CAD build for the part. Positions are in the model's coordinates, mm. Face numbers are marked on the shaded views. A direction names the side the tool comes from. Coordinates: 2 decimals unless noted, no trailing zeros. Loops run counter-clockwise (first coordinate to the right, second up) from the corner with the lowest first, then second, coordinate; pieces in that order, holes last. Notation, with made-up numbers: (7.25, -14) -> (15.25, -14) arc R22 ccw to (15.25, 6) -> close; hole circle Ø8 at (18, -27). An arc over 180 degrees is marked (long way). Write each question's results on one line, items separated by ' | '.
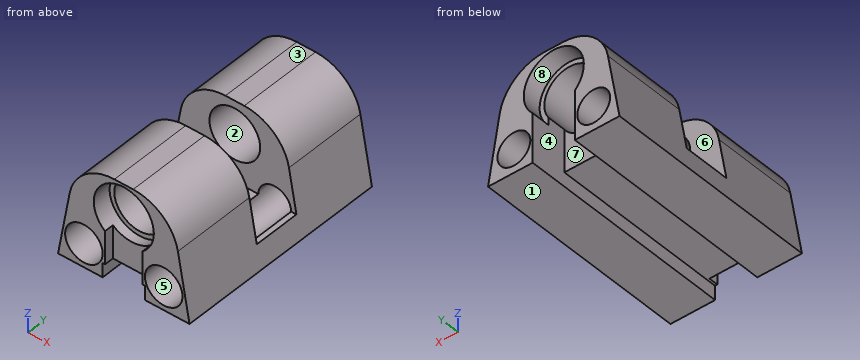
```python
from build123d import *

# Parameters (mm, degrees)
PAD_DEPTH       = 11.5
SKETCH001_W     = 14
SKETCH001_H     = 5
POCKET_DEPTH    = 8.5
SKETCH002_R     = 1.75
POCKET001_DEPTH = 23.001
SKETCH003_R     = 2.7
POCKET002_DEPTH = 23.001
SKETCH004_R     = 2
POCKET003_DEPTH = 5
SKETCH005_W     = 4.5
SKETCH005_H     = 7.5
POCKET004_DEPTH = 4
SKETCH006_W     = 4
SKETCH006_H     = 7.5
POCKET005_DEPTH = 1
SKETCH007_W     = 4.5
SKETCH007_H     = 21
POCKET006_DEPTH = 1.5
SKETCH008_R     = 3.2
POCKET007_DEPTH = 2
SKETCH009_R     = 3.2
POCKET008_DEPTH = 2


with BuildPart() as part:
    # Sketch → Pad (new body, symmetric)
    with BuildSketch(Plane.XZ):
        with BuildLine():
            Line((-7, 0), (7, 0))
            Line((7, 0), (5.766491, 7))
            ThreePointArc((5.766491, 7), (4.111247, 9.867503), (1, 11))
            Line((-1, 11), (1, 11))
            ThreePointArc((-1, 11), (-4.111247, 9.867503), (-5.766491, 7))
            Line((-5.766491, 7), (-7, 0))
        make_face()
    extrude(amount=PAD_DEPTH, both=True)

    # Sketch001 → Pocket (cut)
    with BuildSketch(Plane(origin=(0, 0, 11), x_dir=(-1, 0, 0), z_dir=(0, 0, 1))):
        Rectangle(SKETCH001_W, SKETCH001_H)
    extrude(amount=-POCKET_DEPTH, mode=Mode.SUBTRACT)

    # Sketch002 → Pocket001 (cut, through all)
    with BuildSketch(Plane.XZ.offset(11.5)):
        with Locations((-4.25, 2.5)):
            Circle(SKETCH002_R)
        with Locations((4.25, 2.5)):
            Circle(SKETCH002_R)
    extrude(amount=-POCKET001_DEPTH, mode=Mode.SUBTRACT)

    # Sketch003 → Pocket002 (cut, through all)
    with BuildSketch(Plane.XZ.offset(11.5)):
        with Locations((0, 7.5)):
            Circle(SKETCH003_R)
    extrude(amount=-POCKET002_DEPTH, mode=Mode.SUBTRACT)

    # Sketch004 → Pocket003 (cut)
    with BuildSketch(Plane.XZ.offset(11.5)):
        with Locations((-4.25, 2.5)):
            Circle(SKETCH004_R)
        with Locations((4.25, 2.5)):
            Circle(SKETCH004_R)
    extrude(amount=-POCKET003_DEPTH, mode=Mode.SUBTRACT)

    # Sketch005 → Pocket004 (cut)
    with BuildSketch(Plane(origin=(0, 11.5, 0), x_dir=(1, 0, 0), z_dir=(0, 1, 0))):
        with Locations((0, -3.75)):
            Rectangle(SKETCH005_W, SKETCH005_H)
    extrude(amount=-POCKET004_DEPTH, mode=Mode.SUBTRACT)

    # Sketch006 → Pocket005 (cut)
    with BuildSketch(Plane.XZ.offset(11.5)):
        with Locations((0, 3.75)):
            Rectangle(SKETCH006_W, SKETCH006_H)
    extrude(amount=-POCKET005_DEPTH, mode=Mode.SUBTRACT)

    # Sketch007 → Pocket006 (cut)
    with BuildSketch(Plane(origin=(0, 0, 0), x_dir=(1, 0, 0), z_dir=(0, 0, -1))):
        with Locations((0, 1.5)):
            Rectangle(SKETCH007_W, SKETCH007_H)
    extrude(amount=-POCKET006_DEPTH, mode=Mode.SUBTRACT)

    # Sketch008 → Pocket007 (cut)
    with BuildSketch(Plane(origin=(0, 11.5, 0), x_dir=(1, 0, 0), z_dir=(0, 1, 0))):
        with Locations((0, -7.5)):
            Circle(SKETCH008_R)
    extrude(amount=-POCKET007_DEPTH, mode=Mode.SUBTRACT)

    # Sketch009 → Pocket008 (cut)
    with BuildSketch(Plane.XZ.offset(11.5)):
        with Locations((0, 7.5)):
            Circle(SKETCH009_R)
    extrude(amount=-POCKET008_DEPTH, mode=Mode.SUBTRACT)


solid = part.part
```
Q1. Cut at D-D on y = -0.5. Write the cut outline in (x, z).
Results are:
outline: (-7, 0) -> (-2.25, 0) -> (-2.25, 1.5) -> (2.25, 1.5) -> (2.25, 0) -> (7, 0) -> (6.56, 2.5) -> (6, 2.5) arc R1.75 cw to (2.5, 2.5) -> (-2.5, 2.5) arc R1.75 cw to (-6, 2.5) -> (-6.56, 2.5) -> close
Q2. Pull direction Z, two halves, no side cores. Call the marked faces 1, 2, 3 and 4: +Z half, -Z half, draft (parallel to the pull), parting line (faces both ways), or undercut.
Results are:
face 1: -Z half | face 2: undercut | face 3: +Z half | face 4: draft
Q3. Wall check: L1, parallel to Y at x = 5.25, z = 4; L2, parallel to X at y = 3.5, z = 2.5; L3, parallel to Y at x = -1, z = 4.5. Give the ranges that are in metal, low to high. Write a range as from..to.
Results are:
L1: -6.5..-2.5, 2.5..11.5 | L2: -6.56..-6, -2.5..2.5, 6..6.56 | L3: -9.5..-2.5, 2.5..7.5
Q4. Cut at B-B on x = -4.25. Write the cut outline in (y, z), and give its area (3 significant figures).
Results are:
outline: (-11.5, 0) -> (11.5, 0) -> (11.5, 0.75) -> (-6.5, 0.75) -> (-6.5, 0.5) -> (-11.5, 0.5) -> close; (-11.5, 4.5) -> (-6.5, 4.5) -> (-6.5, 4.25) -> (-2.5, 4.25) -> (-2.5, 9.75) -> (-11.5, 9.75) -> close; (2.5, 4.25) -> (11.5, 4.25) -> (11.5, 9.75) -> (2.5, 9.75) -> close | area: 114 mm^2
Q5. Which spindle directions (+Z, -Z, +X, -X, +Y, -Y) get a long thin tool onto all of the face, cutting with end or side? Do the marked faces 5, 6, 7 and 8. Say none if no direction does.
Results are:
face 5: -Y | face 6: +Z, +X, -X | face 7: -Z, +Y | face 8: +Y
Q6. Cut at A-A on y = 8. Write the cut outline in (x, z).
Results are:
outline: (-7, 0) -> (-2.25, 0) -> (-2.25, 6.01) arc R2.7 cw (long way) to (2.25, 6.01) -> (2.25, 0) -> (7, 0) -> (5.77, 7) arc R4.84 ccw to (1, 11) -> (-1, 11) arc R4.84 ccw to (-5.77, 7) -> close; hole circle Ø3.5 at (-4.25, 2.5); hole circle Ø3.5 at (4.25, 2.5)
Q7. Drop flat-ended pins along their axis: pin 1 (2.5 mm diameter, centred on x = 0, y = 0, fed in from +Z); pin 2 (2 mm diameter, centred on y = 6, z = 3.5, fed in from -X); pin 3 (1.4 mm diameter, centred on x = -1, z = 4.5, fed in from +Y). Give the stop position or say it passes through.
Results are:
pin 1: z = 2.5 | pin 2: x = -6.56 | pin 3: y = 7.5
Q8. Cut at C-C on z = 7.5. Write the cut outline in (x, y).
Results are:
outline: (-5.65, -11.5) -> (-3.2, -11.5) -> (-3.2, -9.5) -> (-2.7, -9.5) -> (-2.7, -2.5) -> (-5.65, -2.5) -> close; (-5.65, 2.5) -> (-2.7, 2.5) -> (-2.7, 9.5) -> (-3.2, 9.5) -> (-3.2, 11.5) -> (-5.65, 11.5) -> close; (2.7, -9.5) -> (3.2, -9.5) -> (3.2, -11.5) -> (5.65, -11.5) -> (5.65, -2.5) -> (2.7, -2.5) -> close; (2.7, 2.5) -> (5.65, 2.5) -> (5.65, 11.5) -> (3.2, 11.5) -> (3.2, 9.5) -> (2.7, 9.5) -> close
